Autodesk Inventor part; units mm, degrees
ref_plane "YZ Plane" through (0, 0, 0) normal (1, 0, 0) x (0, 1, 0)
ref_plane "XZ Plane" through (0, 0, 0) normal (0, 1, 0) x (-1, 0, 0)
ref_plane "XY Plane" through (0, 0, 0) normal (0, 0, 1) x (1, 0, 0)
sketch "Sketch1" plane through (0, 0, 0) normal (0, 0, 1) x (1, 0, 0)
  arc A0 (-1.9, 11.5447) -> (-3.0282, 11.3013) centre (0, 0) ccw construction
  line L0 (0, 7.75) -> (0, 0) construction
  arc A1 (1.9, 11.5447) -> (-1.9, 11.5447) centre (0, 0) ccw construction
  circle A2 centre (0, 0) radius 4.05
  line L1 (11.7, 0) -> (11.7, -20)
  line L2 (11.7, -20) -> (-11.7, -20)
  line L3 (-11.7, -20) -> (-11.7, 0)
  arc A3 (11.7, 0) -> (3.0282, 11.3013) centre (0, 0) ccw
  arc A4 (-11.7, 0) -> (11.7, 0) centre (0, 0) ccw construction
  line L4 (3.0282, 11.3013) -> (1.872, 6.9864)
  line L5 (-1.872, 6.9864) -> (-3.0282, 11.3013)
  arc A5 (-1.872, 6.9864) -> (1.872, 6.9864) centre (0, 7.488) ccw
  arc A6 (3.0282, 11.3013) -> (1.9, 11.5447) centre (0, 0) ccw construction
  arc A7 (-3.0282, 11.3013) -> (-11.7, 0) centre (0, 0) ccw
  line L6 (-1.872, 6.9864) -> (0, 0) construction
  line L7 (0, 0) -> (1.872, 6.9864) construction
  line L8 (0, 5.55) -> (0, 4.05) construction
  dimension "d3" = 8.1
  dimension "d0" = 23.4
  dimension "d4" = 20
  dimension "d8" = 30
  dimension "d9" = 1.5
extrude "Extrusion1" add sketch "Sketch1" along normal blind 3
sketch "Sketch2" plane through (-11.7, -20, 0) normal (-1, 0, 0) x (0, 0, 1)
  line L0 (0, 20) -> (58, 20)
  line L1 (58, 20) -> (58, 0)
  line L2 (58, 0) -> (0, 0)
  line L3 (0, 0) -> (0, 20)
  line L4 (0, 0) -> (3, 0)
  line L5 (3, 20) -> (3, 0)
  dimension "d10" = 55
extrude "Extrusion2" add sketch "Sketch2" along normal blind 3
sketch "Sketch3" plane through (-11.7, -20, 58) normal (0, 0, 1) x (1, 0, 0)
  circle A0 centre (11.7, 20) radius 4.05 construction
  arc A1 (0, 20) -> (23.4, 20) centre (11.7, 20) ccw
  line L0 (23.4, 0) -> (23.4, 20)
  line L1 (23.4, 20) -> (23.4, 0)
  line L2 (23.4, 0) -> (0, 0)
  line L3 (23.4, 0) -> (-3, 0) construction
  line L4 (0, 0) -> (0, 20)
extrude "Extrusion3" add sketch "Sketch3" against normal blind 4
sketch "Sketch4" plane through (-14.7, -20, 58) normal (0, 0, 1) x (1, 0, 0)
  circle A0 centre (8.45, 5) radius 1.35
  circle A1 centre (20.95, 5) radius 1.35
  line L0 (8.45, 5) -> (20.95, 5) construction
  line L1 (14.7, 5) -> (14.7, 20) construction
  dimension "d15" = 12.5
  dimension "d16" = 2.7
  dimension "d17" = 15
extrude "Extrusion4" cut sketch "Sketch4" against normal up to surface (4 mm away)
sketch "Sketch5" plane through (11.7, -20, 0) normal (1, 0, 0) x (0, 0, -1)
  line L0 (0, 31.3013) -> (0, 20) construction
  line L1 (0, 20) -> (-58, 20)
  line L2 (-58, 20) -> (-58, 0)
  line L3 (-58, 0) -> (0, 0)
  line L4 (0, 0) -> (0, 20)
extrude "Extrusion5" add sketch "Sketch5" along normal blind 3
sketch "Sketch7" plane through (-14.7, -20, 58) normal (0, 0, 1) x (1, 0, 0)
  line L0 (0, 20) -> (2.5, 20)
  line L1 (2.5, 20) -> (2.5, 0)
  line L2 (2.5, 0) -> (0, 0)
  line L3 (0, 0) -> (0, 20)
  line L4 (29.4, 20) -> (26.9, 20)
  line L5 (26.9, 20) -> (26.9, 0)
  line L6 (26.9, 0) -> (29.4, 0)
  line L7 (29.4, 0) -> (29.4, 20)
  point P0 (14.7, 20)
  dimension "d27" = 2.5
extrude "Extrusion7" add sketch "Sketch7" along normal blind 3
sketch "Sketch6" plane through (14.7, -20, 0) normal (1, 0, 0) x (0, 0, -1)
  line L0 (-45.5, 10) -> (-15.5, 10) construction
  line L1 (-58, 0) -> (0, 0) construction
  circle A0 centre (-45.5, 10) radius 2.8813
  circle A1 centre (-15.5, 10) radius 2.8813
  line L2 (0, 20) -> (-61, 20) construction
  line L3 (-30.5, 20) -> (-30.5, 10) construction
  dimension "d22" = 30
  dimension "d23" = 5.7625
  dimension "d24" = 10
extrude "Extrusion6" cut sketch "Sketch6" against normal through all
sketch "Sketch8" plane through (14.7, -20, 0) normal (1, 0, 0) x (0, 0, -1)
  circle A0 centre (-15.5, 10) radius 5
  circle A1 centre (-45.5, 10) radius 5
  circle A2 centre (-15.5, 10) radius 2.8813 construction
  circle A3 centre (-45.5, 10) radius 2.8813 construction
  point P0 (0, 20)
  dimension "d30" = 10
extrude "Extrusion8" cut sketch "Sketch8" against normal blind 3
properties part number "Xgantry_CableChain_top_connector"
Can you work these out from the model? Positions are in its coordinate system, mm. A direction names the side the tool comes from. Round coordinates to 2 decimals unless told otherwise and drop trailing zeros. Order: outer loops, then holes, each group sorted by start corner. A loop starts at its lowest first (then second) coordinate and runs counter-clockwise, first axis right, second up.
(1) We'd pull the mould along Z, two halves only. Please class faces 5 (the face through (0, -8, 0)), 6 (the face through (13.221, -9.78, 20.495)), 7 (the face through (-0.878, 3.954, 1.479)), 8 (the face through (0, -14, 54)): +Z half, -Z half, draft (parallel to the pull), parting line (faces both ways), or undercut.
Results are:
face 5: -Z half
face 6: undercut
face 7: draft
face 8: undercut
(2) I'm going to push flat-ended pins straight in: pin 1 (6.5 mm diameter, centred on y = -10, z = 15.5, fed in from +X); pin 2 (1.6 mm diameter, centred on x = -6.25, y = -15, fed in from +Z); pin 3 (3.5 mm diameter, centred on x = -13, z = 39.5, fed in from +Y). Where does each tip first touch, or does it pass through?
Results are:
pin 1: stops at x = -11.7
pin 2: stops at z = 3
pin 3: stops at y = 0
(3) If we section it at C-C (z = 15.5): Please give me the cut outline in (x, y).
Results are:
outline: (-14.7, -20) - (-11.7, -20) - (-11.7, -12.88) - (-14.7, -12.88) - close; (-14.7, -7.12) - (-11.7, -7.12) - (-11.7, 0) - (-14.7, 0) - close; (11.7, -20) - (14.7, -20) - (14.7, -15) - (11.7, -15) - close; (11.7, -5) - (14.7, -5) - (14.7, 0) - (11.7, 0) - close
(4) If we section it at B-B (x = 0): Please give me the cut outline in (y, z), plus the area to 4 significant figures.
Results are:
outline: (-20, 0) - (-4.05, 0) - (-4.05, 3) - (-20, 3) - close; (-20, 54) - (-11.7, 54) - (-11.7, 58) - (-20, 58) - close; (4.05, 0) - (5.55, 0) - (5.55, 3) - (4.05, 3) - close
area: 85.55 mm2
(5) If we section it at A-A (z = 52): Please give me the cut outline in (x, y), plus the area to 3 significant figures.
Results are:
outline: (-14.7, -20) - (-11.7, -20) - (-11.7, 0) - (-14.7, 0) - close; (11.7, -20) - (14.7, -20) - (14.7, 0) - (11.7, 0) - close
area: 120 mm2
(6) If I drill on L1, parallel to Y at x = 12.5, z = 15.5; L2, parallel to X at y = -15, z = 58.5; L3, parallel to X at y = -16, z = 23.5, over which ranges is the centre line in solid material (lowest first)?
Results are:
L1: y = -20 to -15, -5 to 0
L2: x = -14.7 to -12.2, 12.2 to 14.7
L3: x = -14.7 to -11.7, 11.7 to 14.7
(7) On a 3-axis mill with a long thin cutter (end or side, diameter ignored), from which of +Z, -Z, +X, -X, +Y, -Y can I reach the whole of each face in a straight line? I mean faces 1 (the face through (6.074, -13.661, 56.028)), 2 (the face through (-0.257, -11.697, 56.028)), 3 (the face through (-2.44, 9.11, 1.48)), 4 (the face through (-11.7, -10, 28)). Say none if no direction works.
Results are:
face 1: +Z
face 2: +Z, +Y
face 3: +Z, -Z, +Y
face 4: +Y, -Y
(8) If we section it at D-D (y = 8.5): Please give me the cut outline in (x, z).
Results are:
outline: (-8.04, 0) - (-2.28, 0) - (-2.28, 3) - (-8.04, 3) - close; (2.28, 0) - (8.04, 0) - (8.04, 3) - (2.28, 3) - close
